Geometry check sheet. Reference: drawing and pictorial views, mm from the part's lowest x, y, z. A direction names the side the tool comes from. Give positions to 0.01 mm unless a question says otherwise; leave off trailing zeros. Loops run counter-clockwise (first coordinate to the right, second up) from the corner with the lowest first, then second, coordinate; pieces in that order, holes last. Notation, with made-up numbers: (-26.5, 72.25) - (9.5, 72.25) arc R22 ccw to (9.5, 108.25) - close; hole circle Ø3 at (-36.75, -7). An arc over 180 degrees is marked (long way). Answer in a Markdown table with one row per item. Add a question column.
(1) Sectioned sample at B-B on x = 12. Enter the section's corners in (y, z).
(2) Sectioned sample at A-A on z = 0.6. State how many separate pieces and enclosed holes the cut face has, then the cut area to 3 significant figures.
(3) Thickness scan on L1, parallel to Y at x = 24.5, z = 2.1; L2, parallel to X at y = 26.5, z = 0.25; L3, parallel to Y at x = 44.5, z = 2.7. Record the ranges inside material, lowest first.
(4) Draft check along Y on the marked faces 6, 7, 8 and 9. Enter one of: released by +Y, released by -Y, zero draft, split by the parting line, or undercut.
(5) Sectioned sample at D-D on y = 41.5. Enter the section's corners in (x, z), then the cut area to 3 significant figures.
(6) Go/stop test with flat-tipped pins: P1, Ø0.9, axis at x = 7, z = 1.5, coming from the +Y side; P2, Ø1.5, axis at y = 6.5, z = 2, coming from the -X side; P3, Ø3.5, axis at x = 24.5, y = 15, coming from the +Z side; P4, Ø1.5, axis at y = 8, z = 2, coming from the +X side. Record where each tip stops, or that it passes through.
(7) Set-up check for the marked faces 1, 2, 3, 4 and 5: record each of +Z, -Z, +X, -X, +Y, -Y from which the full face is reachable in a straight line by a thin tool's end or side.
(8) Sectioned sample at C-C on y = 34. Enter the section's corners in (x, z), then the cut area to 3 significant figures.
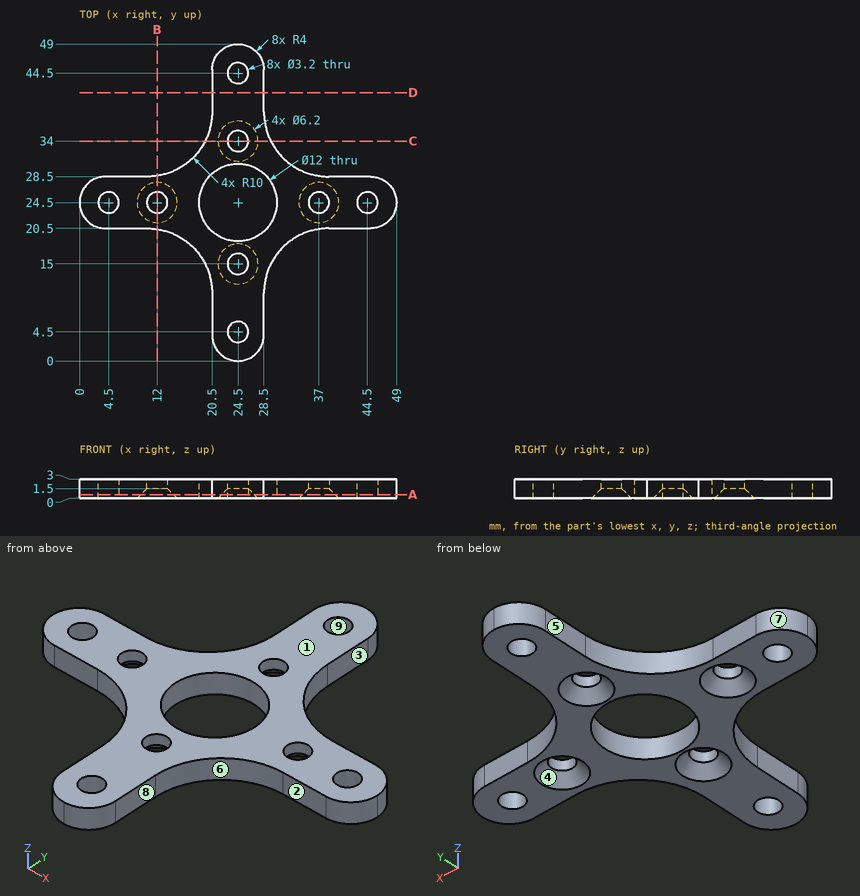
Reply:
| question | item | result |
|---|---|---|
| 1 | outline | (20.39, 0) - (21.4, 0) - (22.9, 1.5) - (22.9, 3) - (20.39, 3) - close; (26.1, 1.5) - (27.6, 0) - (28.61, 0) - (28.61, 3) - (26.1, 3) - close |
| 2 | separate pieces | 1 |
| 2 | enclosed holes | 9 |
| 2 | area | 555 mm^2 |
| 3 | L1 | 0 to 2.9, 6.1 to 13.4, 16.6 to 18.5, 30.5 to 32.4, 35.6 to 42.9, 46.1 to 49 |
| 3 | L2 | 0.54 to 9.97, 14.03 to 18.84, 30.16 to 34.97, 39.03 to 48.46 |
| 3 | L3 | 20.5 to 22.9, 26.1 to 28.5 |
| 4 | face 6 | released by -Y |
| 4 | face 7 | released by +Y |
| 4 | face 8 | zero draft |
| 4 | face 9 | undercut |
| 5 | outline | (20.5, 0) - (28.5, 0) - (28.5, 3) - (20.5, 3) - close |
| 5 | area | 24.0 mm^2 |
| 6 | P1 | y = 28.5 |
| 6 | P2 | x = 20.5 |
| 6 | P3 | z = 3 |
| 6 | P4 | x = 28.5 |
| 7 | face 1 | +Z, +X, -X, +Y, -Y |
| 7 | face 2 | +Z, -Z, +X, -Y |
| 7 | face 3 | +Z, -Z, +X, +Y |
| 7 | face 4 | -Z |
| 7 | face 5 | +Z, -Z, -X, +Y |
| 8 | outline | (19.43, 0) - (21.4, 0) - (22.9, 1.5) - (22.9, 3) - (19.43, 3) - close; (26.1, 1.5) - (27.6, 0) - (29.57, 0) - (29.57, 3) - (26.1, 3) - close |
| 8 | area | 18.6 mm^2 |
